Work out the finished part from the listing and answer in its coordinate system (mm). A direction names the side the tool comes from. Round coordinates to 2 decimals unless told otherwise and drop trailing zeros. Order: outer loops, then holes, each group sorted by start corner. A loop starts at its lowest first (then second) coordinate and runs counter-clockwise, first axis right, second up. Notation, with made-up numbers: (-31, 72) - (-12, 72) arc R27 cw to (-12, 107) - close; hole circle Ø6 at (-36, 9). An arc over 180 degrees is marked (long way). Answer in a Markdown table with one row per item.
from build123d import *

# Parameters (mm, degrees)
SKETCH1_W           = 1000
SKETCH1_H           = 1567.75
SKETCH1_W_2         = 940
SKETCH1_H_2         = 1507.75
BOSS_EXTRUDE1_DEPTH = 15
SKETCH2_W           = 26
SKETCH2_H           = 26


with BuildPart() as part:
    # Sketch1 → Boss-Extrude1 (new body, symmetric)
    with BuildSketch(Plane.XY):
        Rectangle(SKETCH1_W, SKETCH1_H)
        Rectangle(SKETCH1_W_2, SKETCH1_H_2, mode=Mode.SUBTRACT)
    extrude(amount=BOSS_EXTRUDE1_DEPTH, both=True)

    # Cut-Sweep1: sweep along a path in Sketch4
    with BuildLine(Plane.XY) as cut_sweep1_path:
        Line((-485, 768.875), (-485, -768.875))
        Line((-485, -768.875), (485, -768.875))
        Line((485, -768.875), (485, 768.875))
        Line((485, 768.875), (-485, 768.875))
    # Sketch2 → Cut-Sweep1 (sweep, cut)
    with BuildSketch(Plane(origin=(0, 0, 0), x_dir=(0, 0, -1), z_dir=(1, 0, 0))):
        with Locations((0, 768.875)):
            Rectangle(SKETCH2_W, SKETCH2_H)
    sweep(path=cut_sweep1_path.line, transition=Transition.RIGHT, mode=Mode.SUBTRACT)

    # Sketch7 → Revolve1 (revolve)
    with BuildSketch(Plane.XY):
        with BuildLine():
            Line((-340, 783.875), (-340, 788.875))
            Line((-340, 788.875), (-345, 788.875))
            ThreePointArc((-345, 788.875), (-342.5, 786.375), (-345, 783.875))
            Line((-345, 783.875), (-340, 783.875))
        make_face()
    revolve1 = revolve(axis=Axis((-340, 795.104340353, 0), (0, 1, 0)))

    # Mirror1: Revolve1 across plane
    add(revolve1.mirror(Plane(origin=(0, 0, 0), x_dir=(0, 0, 1), z_dir=(1, 0, 0))))


solid = part.part
1) Which of the six approach directions +Z, -Z, +X, -X, +Y, -Y give full straight-line access (tool end or side, diameter ignored) to faces 4 (the face through (-7, 753.875, 0)), 5 (the face through (477, -235, 13)), 6 (the face through (-484, 236, -15))?
Filled in:
| item | result |
|---|---|
| face 4 | +Z, -Z |
| face 5 | none |
| face 6 | -Z, +X, -X, +Y, -Y |
2) This flat-tipped pin is pushed along its axis until it touches: pin 1 (2 mm diameter, centred on x = 146, z = -5.5, fed in from +Y) (3 decimals). Where does it stop, or does it pass through?
Filled in:
| item | result |
|---|---|
| pin 1 | stops at y = 783.875 |
3) Find section B-B, the plane x = 158. Give the vertices of the cut face in (y, z) (3 decimals).
Filled in:
| item | result |
|---|---|
| outline | (-783.875, -15) - (-753.875, -15) - (-753.875, 15) - (-783.875, 15) - close; (753.875, -15) - (783.875, -15) - (783.875, 15) - (753.875, 15) - close; hole (-781.875, -13) - (-755.875, -13) - (-755.875, 13) - (-781.875, 13) - close; hole (755.875, -13) - (781.875, -13) - (781.875, 13) - (755.875, 13) - close |
4) Find section A-A, the plane y = 82. Give the vertices of the cut face in (x, z), then the cut area to 3 significant figures.
Filled in:
| item | result |
|---|---|
| outline | (-500, -15) - (-470, -15) - (-470, 15) - (-500, 15) - close; (470, -15) - (500, -15) - (500, 15) - (470, 15) - close; hole (-498, -13) - (-472, -13) - (-472, 13) - (-498, 13) - close; hole (472, -13) - (498, -13) - (498, 13) - (472, 13) - close |
| area | 448 mm^2 |
5) The mould has two halves that part along Z. Classify faces 1 (the face through (-477, -235, -13)), 2 (the face through (500, -11, 0)), 3 (the face through (-484, 236, 15)): released by +Z, released by -Z, zero draft, split by the parting line, or undercut.
Filled in:
| item | result |
|---|---|
| face 1 | undercut |
| face 2 | zero draft |
| face 3 | released by +Z |
6) Find the intervals of material crossed by probe 1 along X at (y, z) = (-32, -10.25); probe 2 along Y at (x, z) = (-135, -6.5) (3 decimals); probe 3 along Y at (x, z) = (-422.5, -13.5) (3 decimals), in increasing order. Write a range as from..to.
Filled in:
| item | result |
|---|---|
| probe 1 | x = -500..-498, -472..-470, 470..472, 498..500 |
| probe 2 | y = -783.875..-781.875, -755.875..-753.875, 753.875..755.875, 781.875..783.875 |
| probe 3 | y = -783.875..-753.875, 753.875..783.875 |
